from build123d import *

# Parameters (mm, degrees)
EXTRUDE_THIN1_DEPTH = 16
CUT_EXTRUDE1_DEPTH  = 10
BOSS_EXTRUDE1_START = -1.5
BOSS_EXTRUDE1_DEPTH = 1.5


with BuildPart() as part:
    # Sketch1 → Extrude-Thin1 (new body)
    with BuildSketch(Plane.XY):
        with BuildLine():
            Line((-15, 26), (-15, 0))
            Line((-15, 0), (15, 0))
            Line((15, 0), (15, 26))
            ThreePointArc((15, 26), (0, 41), (-15, 26))
        make_face()
        with BuildLine():
            Line((-14, 26), (-14, 1))
            Line((-14, 1), (14, 1))
            Line((14, 1), (14, 26))
            ThreePointArc((14, 26), (0, 40), (-14, 26))
        make_face(mode=Mode.SUBTRACT)
    extrude(amount=EXTRUDE_THIN1_DEPTH)

    # Sketch2 → Cut-Extrude1 (cut)
    with BuildSketch(Plane(origin=(0, 0, 0), x_dir=(-1, 0, 0), z_dir=(0, -1, 0))):
        with BuildLine():
            Line((3, -7), (3, 0))
            Line((3, 0), (-3, 0))
            Line((-3, 0), (-3, -7))
            ThreePointArc((-3, -7), (0, -10), (3, -7))
        make_face()
    extrude(amount=-CUT_EXTRUDE1_DEPTH, mode=Mode.SUBTRACT)

    # Sketch3 → Boss-Extrude1 (add)
    with BuildSketch(Plane.XY.offset(16).offset(BOSS_EXTRUDE1_START)):
        with BuildLine():
            Line((-15, 0), (15, 0))
            Line((15, 0), (15, 26))
            ThreePointArc((15, 26), (0, 41), (-15, 26))
            Line((-15, 26), (-15, 0))
        make_face()
    extrude(amount=BOSS_EXTRUDE1_DEPTH)


solid = part.part
Input: part model. Units: mm. Frame: model coordinates. A direction names the side the tool comes from. Coordinates: 2 decimals unless noted, no trailing zeros. Loops run counter-clockwise (first coordinate to the right, second up) from the corner with the lowest first, then second, coordinate; pieces in that order, holes last.
(1) Section A-A on z = 13. Return the cut outline in (x, y), then the cut area to 3 significant figures.
(2) Set-up query: faces 4 (the face through (3, 0.5, 3.5)), 5 (the face through (-4, 0, 8)), 6 (the face through (14, 13, 7)). Return all of +Z, -Z, +X, -X, +Y, -Y with unobstructed straight access to the full face (end or side cutting, diameter ignored); none if empty.
(3) Material intervals for probe 1 along X at (y, z) = (4.5, 3.5); probe 2 along Z at (x, y) = (-1, 16.5); probe 3 along Y at (x, z) = (-0.25, 5), sorted ascending.
(4) Pull-direction query (Y, two-part tool) for faces 1 (the face through (-14, 14, 7)), 2 (the face through (0, 21, 16)), 3 (the face through (0, 41, 8)); classes: released by +Y, released by -Y, zero draft, split by the parting line, or undercut.
(5) Section C-C on x = 0. Return the cut outline in (y, z), then the cut area to 3 significant figures.
(6) Section B-B on y = 19.5. Return the cut outline in (x, z).
(7) Section D-D on z = 4.5. Return the cut outline in (x, y), then the cut area to 3 significant figures.
(8) First-contact query: pin 1 Ø3 at (x, y) = (-12, 23.5) entering from -Z; pin 2 Ø1 at (x, z) = (-4, 11.5) entering from +Y. Flat tips, straight axial feed; report the tip coordinate or a pass-through.
Data:
1. outline: (-15, 0) - (15, 0) - (15, 26) arc R15 ccw to (-15, 26) - close; hole (-14, 1) - (14, 1) - (14, 26) arc R14 ccw to (-14, 26) - close
1. area: 126 mm2
2. face 4: -Z, -Y
2. face 5: +Z, -Z, +X, -X, -Y
2. face 6: -Z
3. probe 1: x = -15 to -14, 14 to 15
3. probe 2: z = 14.5 to 16
3. probe 3: y = 40 to 41
4. face 1: undercut
4. face 2: zero draft
4. face 3: released by +Y
5. outline: (0, 10) - (1, 10) - (1, 14.5) - (40, 14.5) - (40, 0) - (41, 0) - (41, 16) - (0, 16) - close
5. area: 80.5 mm2
6. outline: (-15, 0) - (-14, 0) - (-14, 14.5) - (14, 14.5) - (14, 0) - (15, 0) - (15, 16) - (-15, 16) - close
7. outline: (-15, 0) - (-3, 0) - (-3, 1) - (-14, 1) - (-14, 26) arc R14 cw to (14, 26) - (14, 1) - (3, 1) - (3, 0) - (15, 0) - (15, 26) arc R15 ccw to (-15, 26) - close
7. area: 120 mm2
8. pin 1: stops at z = 14.5
8. pin 2: stops at y = 40.59
